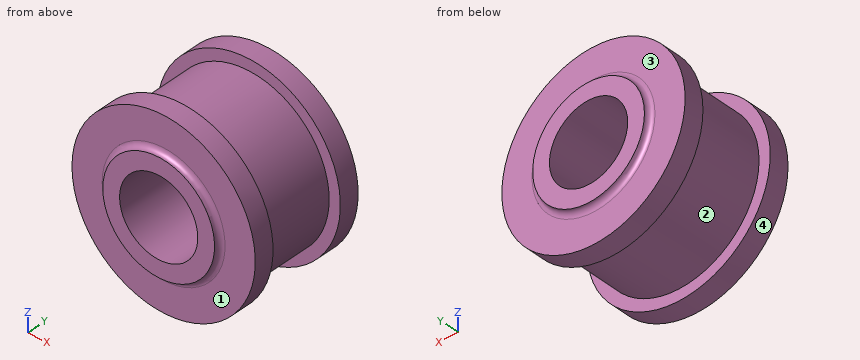
```python
from build123d import *

# Parameters (mm, degrees)
CUT_EXTRUDE1_REACH = 83.308
SKETCH2_R          = 17.5
FILLET1_R          = 2.5


with BuildPart() as part:
    # Sketch1 → Revolve1 (revolve)
    with BuildSketch(Plane.XY, mode=Mode.PRIVATE) as revolve1_sk:
        Polygon((0, 0), (25, 0), (25, 2.5), (41, 2.5), (41, 11.5), (36, 11.5), (36, 45.5), (41, 45.5), (41, 54.5), (25, 54.5), (25, 57), (0, 57), align=None)
    revolve(revolve1_sk.sketch.rotate(Axis((0, 60.737704918, 0), (0, -1, 0)), 180), axis=Axis((0, 60.737704918, 0), (0, -1, 0)))

    # Sketch2 → Cut-Extrude1 (cut, up to next)
    with BuildSketch(Plane(origin=(0, 57, 0), x_dir=(1, 0, 0), z_dir=(0, 1, 0)), mode=Mode.PRIVATE) as cut_extrude1_sk1:
        with Locations(Location((0, 0, 0), (0, 0, 180))):
            Circle(SKETCH2_R)
    cut_extrude1_tool1 = extrude(cut_extrude1_sk1.sketch, amount=-CUT_EXTRUDE1_REACH, mode=Mode.PRIVATE) & part.part
    add(cut_extrude1_tool1.solids().sort_by_distance((0, 57, 0))[0], mode=Mode.SUBTRACT)

    # Fillet1
    fillet1_edges = [part.edges().sort_by_distance(p)[0] for p in [
        (25, 54.5, 0),
        (25, 2.5, 0),
    ]]
    fillet(fillet1_edges, radius=FILLET1_R - 0.0001)  # a hair under: the kernel refuses the full size


solid = part.part
```
Geometry: final body of the model. Coordinates: model frame, mm. Face numbers are marked on the shaded views. Give positions to 0.01 mm unless a question says otherwise; leave off trailing zeros. Write each loop counter-clockwise with the first axis right and the second up, starting at its lowest first coordinate (ties: lowest second). Pieces come first, ordered by that corner, then holes.
1. Section query C-C, the plane y = 53. Return loops of the section in (x, z).
2. Line query: probe 1 along Z at (x, y) = (0, 14); probe 2 along Y at (x, z) = (-38, -7.5); probe 3 along Y at (x, z) = (30.5, -3). Output: solid intervals per line, ascending.
3. Section query D-D, the plane z = 31.5. Return loops of the section in (x, y).
4. Draft query along Y for the marked faces 1, 2, 3 and 4. Return one class per face: released by +Y, released by -Y, zero draft, split by the parting line, or undercut.
5. Pin query (flat end, axial travel): P1, Ø5, axis at x = 14, y = 26, coming from the -Z side; P2, Ø24.5, axis at x = -4.5, z = 15.5, coming from the +Y side; P3, Ø8, axis at x = -32, z = 16.5, coming from the -Y side; P4, Ø5, axis at x = 15, z = -27, coming from the +Y side. Return the tip coordinate at first contact, or that it passes through.
Computed:
1. outline: circle Ø82 at (0, 0); hole circle Ø35 at (0, 0)
2. probe 1: z = -36 to -17.5, 17.5 to 36
2. probe 2: y = 2.5 to 11.5, 45.5 to 54.5
2. probe 3: y = 2.5 to 54.5
3. outline: (-26.24, 2.5) - (26.24, 2.5) - (26.24, 11.5) - (17.43, 11.5) - (17.43, 45.5) - (26.24, 45.5) - (26.24, 54.5) - (-26.24, 54.5) - (-26.24, 45.5) - (-17.43, 45.5) - (-17.43, 11.5) - (-26.24, 11.5) - close
4. face 1: released by -Y
4. face 2: undercut
4. face 3: released by +Y
4. face 4: zero draft
5. P1: stops at z = -34.11
5. P2: stops at y = 57
5. P3: stops at y = 2.5
5. P4: stops at y = 54.5
